Source: three-view drawing plus pictorial views. Frame: mm from the lowest corner of the part. Round coordinates to 2 decimals unless told otherwise and drop trailing zeros. Order: outer loops, then holes, each group sorted by start corner. A loop starts at its lowest first (then second) coordinate and runs counter-clockwise, first axis right, second up. Notation, with made-up numbers: (-13, -2) -> (11, -2) arc R9 ccw to (11, 4) -> close; hole circle Ø8 at (11, 24.25). An arc over 180 degrees is marked (long way). Use a Markdown table: item, result.
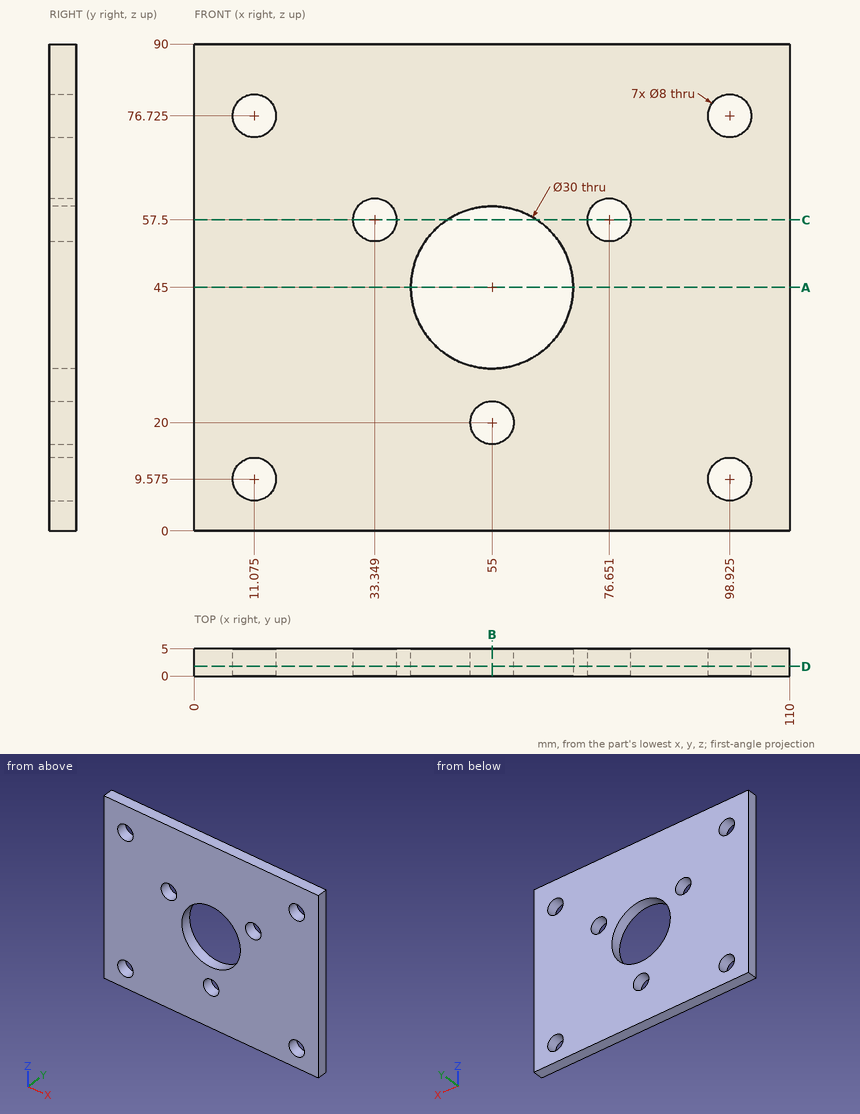
1) Cut plane C-C on z = 57.5. Return loops of the section in (x, y).
Results found:
| item | result |
|---|---|
| outline | (0, 0) -> (29.35, 0) -> (29.35, 5) -> (0, 5) -> close; (37.35, 0) -> (46.71, 0) -> (46.71, 5) -> (37.35, 5) -> close; (63.29, 0) -> (72.65, 0) -> (72.65, 5) -> (63.29, 5) -> close; (80.65, 0) -> (110, 0) -> (110, 5) -> (80.65, 5) -> close |
2) Line query: L1, parallel to Z at x = 55, y = 1.95; L2, parallel to X at y = 2.65, z = 57.5; L3, parallel to X at y = 1.5, z = 11. Output: solid intervals per line, ascending. Write a range as [from, to].
Results found:
| item | result |
|---|---|
| L1 | z = [0, 16], [24, 30], [60, 90] |
| L2 | x = [0, 29.35], [37.35, 46.71], [63.29, 72.65], [80.65, 110] |
| L3 | x = [0, 7.34], [14.81, 95.19], [102.66, 110] |
3) Cut plane B-B on x = 55. Return loops of the section in (y, z), and give its area (3 significant figures).
Results found:
| item | result |
|---|---|
| outline | (0, 0) -> (5, 0) -> (5, 16) -> (0, 16) -> close; (0, 24) -> (5, 24) -> (5, 30) -> (0, 30) -> close; (0, 60) -> (5, 60) -> (5, 90) -> (0, 90) -> close |
| area | 260 mm² |
4) Cut plane A-A on z = 45. Return loops of the section in (x, y), and give its area (3 significant figures).
Results found:
| item | result |
|---|---|
| outline | (0, 0) -> (40, 0) -> (40, 5) -> (0, 5) -> close; (70, 0) -> (110, 0) -> (110, 5) -> (70, 5) -> close |
| area | 400 mm² |
5) Cut plane D-D on y = 1.8. Count the separate pieces of the cut face and the enclosed holes in it, and give its area (3 significant figures).
Results found:
| item | result |
|---|---|
| separate pieces | 1 |
| enclosed holes | 8 |
| area | 8,840 mm² |
